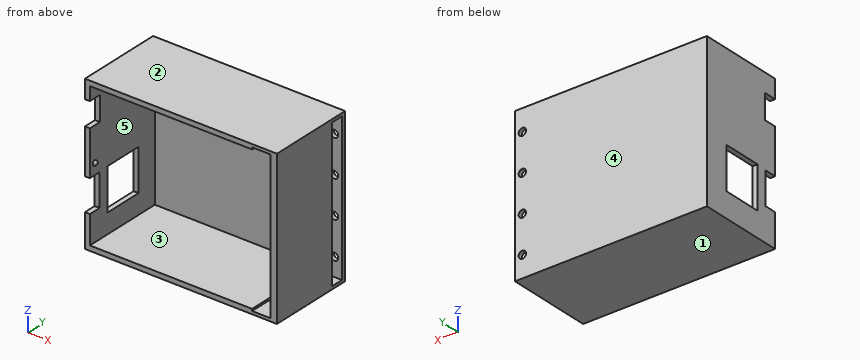
```python
from build123d import *

# Parameters (mm, degrees)
SKETCH1_W           = 77.9
SKETCH1_H           = 62.4
BOSS_EXTRUDE1_DEPTH = 35
SKETCH4_W           = 73.9
SKETCH4_H           = 58.4
CUT_EXTRUDE1_DEPTH  = 33.39
SKETCH7_W           = 13.133474477
SKETCH7_H           = 5
CUT_EXTRUDE6_DEPTH  = 15
SKETCH11_W          = 9.956525523
SKETCH11_H          = 5.15
CUT_EXTRUDE8_DEPTH  = 10
SKETCH12_W          = 17
SKETCH12_H          = 16
CUT_EXTRUDE9_DEPTH  = 10
SKETCH14_W          = 60
SKETCH14_H          = 5
CUT_EXTRUDE10_DEPTH = 10
CUT_EXTRUDE12_START = -33.39
SKETCH16_W          = 9.076585482
SKETCH16_H          = 60
CUT_EXTRUDE12_DEPTH = 33.39
SKETCH15_R          = 1.5
CUT_EXTRUDE11_DEPTH = 10
SKETCH18_W          = 1.605745829
SKETCH18_H          = 60
BOSS_EXTRUDE2_DEPTH = 10


with BuildPart() as part:
    # Sketch1 → Boss-Extrude1 (new body)
    with BuildSketch(Plane(origin=(0, 0, 0), x_dir=(1, 0, 0), z_dir=(0, 1, 0))):
        with Locations((38.95, 31.2)):
            Rectangle(SKETCH1_W, SKETCH1_H)
    extrude(amount=BOSS_EXTRUDE1_DEPTH)

    # Sketch4 → Cut-Extrude1 (cut)
    with BuildSketch(Plane.XZ):
        with Locations((38.95, -31.2)):
            Rectangle(SKETCH4_W, SKETCH4_H)
    extrude(amount=-CUT_EXTRUDE1_DEPTH, mode=Mode.SUBTRACT)

    # Sketch7 → Cut-Extrude6 (cut)
    with BuildSketch(Plane.ZY):
        with Locations((-42.333262762, 2.5)):
            Rectangle(SKETCH7_W, SKETCH7_H)
    extrude(amount=-CUT_EXTRUDE6_DEPTH, mode=Mode.SUBTRACT)

    # Sketch11 → Cut-Extrude8 (cut)
    with BuildSketch(Plane.ZY):
        with Locations((-12.508262762, 2.575)):
            Rectangle(SKETCH11_W, SKETCH11_H)
    extrude(amount=-CUT_EXTRUDE8_DEPTH, mode=Mode.SUBTRACT)

    # Sketch12 → Cut-Extrude9 (cut)
    with BuildSketch(Plane.ZY):
        with Locations((-43.9, 17)):
            Rectangle(SKETCH12_W, SKETCH12_H)
    extrude(amount=-CUT_EXTRUDE9_DEPTH, mode=Mode.SUBTRACT)

    # Sketch14 → Cut-Extrude10 (cut)
    with BuildSketch(Plane(origin=(77.9, 0, 0), x_dir=(0, 0, -1), z_dir=(1, 0, 0))):
        with Locations((31.2, 30.89)):
            Rectangle(SKETCH14_W, SKETCH14_H)
    extrude(amount=-CUT_EXTRUDE10_DEPTH, mode=Mode.SUBTRACT)

    # Sketch16 → Cut-Extrude12 (cut)
    with BuildSketch(Plane(origin=(0, 0, 0), x_dir=(-1, 0, 0), z_dir=(0, -1, 0)).offset(CUT_EXTRUDE12_START)):
        with Locations((-72.361707259, 31.2)):
            Rectangle(SKETCH16_W, SKETCH16_H)
    extrude(amount=CUT_EXTRUDE12_DEPTH, mode=Mode.SUBTRACT)

    # Sketch15 → Cut-Extrude11 (cut)
    with BuildSketch(Plane(origin=(0, 33.39, 0), x_dir=(-1, 0, 0), z_dir=(0, -1, 0))):
        with Locations(Location((-74.9, 8.7, 0), (0, 0, 90))):
            Circle(SKETCH15_R)
        with Locations(Location((-74.9, 23.7, 0), (0, 0, 90))):
            Circle(SKETCH15_R)
        with Locations(Location((-74.9, 38.7, 0), (0, 0, 90))):
            Circle(SKETCH15_R)
        with Locations(Location((-74.9, 53.7, 0), (0, 0, 90))):
            Circle(SKETCH15_R)
    extrude(amount=-CUT_EXTRUDE11_DEPTH, mode=Mode.SUBTRACT)

    # Sketch18 → Boss-Extrude2 (add)
    with BuildSketch(Plane(origin=(0, 0, 0), x_dir=(-1, 0, 0), z_dir=(0, -1, 0))):
        with Locations((-76.097127086, 31.2)):
            Rectangle(SKETCH18_W, SKETCH18_H)
    extrude(amount=-BOSS_EXTRUDE2_DEPTH)

    # Sketch19 → Revolve2 (revolve)
    with BuildSketch(Plane.ZY.offset(-75.294254171)):
        with BuildLine():
            Line((-31.2, 3.5), (-31.2, 1.5))
            ThreePointArc((-31.2, 1.5), (-30.2, 2.5), (-31.2, 3.5))
        make_face()
    revolve(axis=Axis((75.294254171, 3.5, -31.2), (0, -1, 0)))

    # Sketch17 → Revolve4 (revolve)
    with BuildSketch(Plane.ZY.offset(-2)):
        with BuildLine():
            ThreePointArc((-31.2, 3.5), (-32.2, 2.5), (-31.2, 1.5))
            Line((-31.2, 1.5), (-31.2, 3.5))
        make_face()
    revolve(axis=Axis((2, 3.5, -31.2), (0, -1, 0)))


solid = part.part
```
Geometry check sheet. Reference: the model listing, model coordinates, mm. Face numbers are marked on the shaded views. A direction names the side the tool comes from. Round coordinates to 2 decimals unless told otherwise and drop trailing zeros. Loops run counter-clockwise (first coordinate to the right, second up) from the corner with the lowest first, then second, coordinate; pieces in that order, holes last. Notation, with made-up numbers: (73.25, -31.75) - (91.25, -31.75) arc R20 ccw to (91.25, 7.25) - close; hole circle Ø4 at (42, 31.25). An arc over 180 degrees is marked (long way). Use a Markdown table: item, result.
Q1. Cross-section at B-B on z = -8.7. Record the cut outline in (x, y).
Solutions:
| item | result |
|---|---|
| outline | (0, 5.15) - (2, 5.15) - (2, 33.39) - (73.4, 33.39) - (73.4, 35) - (0, 35) - close; (75.29, 0) - (77.9, 0) - (77.9, 28.39) - (76.9, 28.39) - (76.9, 10) - (75.29, 10) - close; (76.4, 33.39) - (77.9, 33.39) - (77.9, 35) - (76.4, 35) - close |
Q2. Draft check along Z on the marked faces 1, 2 and 3. Enter one of: released by +Z, released by -Z, zero draft, split by the parting line, or undercut.
Solutions:
| item | result |
|---|---|
| face 1 | released by -Z |
| face 2 | released by +Z |
| face 3 | undercut |
Q3. Access from +Z, -Z, +X, -X, +Y, -Y to the whole of each face (thin tool, end or side, straight path). Record for the marked faces 4 and 5.
Solutions:
| item | result |
|---|---|
| face 4 | +Z, -Z, +X, -X, +Y |
| face 5 | none |
Q4. Go/stop test with flat-tipped pins: P1, Ø1, axis at x = 48.5, z = -12.5, coming from the -Y side; P2, Ø0.6, axis at x = 1.5, z = -44.5, coming from the -Y side; P3, Ø1.6, axis at x = 1.5, z = -13, coming from the -Y side. Record where each tip stops, or that it passes through.
Solutions:
| item | result |
|---|---|
| P1 | stops at y = 33.39 |
| P2 | stops at y = 5 |
| P3 | stops at y = 5.15 |
Q5. Cross-section at C-C on y = 29.5. Record the cut outline in (x, z).
Solutions:
| item | result |
|---|---|
| outline | (0, -62.4) - (77.9, -62.4) - (77.9, -61.2) - (67.82, -61.2) - (67.82, -60.4) - (2, -60.4) - (2, -2) - (67.82, -2) - (67.82, -1.2) - (77.9, -1.2) - (77.9, 0) - (0, 0) - close |
Q6. Material ranges on line 1 (Z direction, x = 74.9, y = 34.15); line 2 (Z direction, x = 71, y = 27.5); line 3 (X direction, y = 25.5, z = -57.5), recorded low to high.
Solutions:
| item | result |
|---|---|
| line 1 | z = -62.4 to -55.2, -52.2 to -40.2, -37.2 to -25.2, -22.2 to -10.2, -7.2 to 0 |
| line 2 | z = -62.4 to -61.2, -1.2 to 0 |
| line 3 | x = 0 to 2, 76.9 to 77.9 |
Q7. Cross-section at A-A on z = -38.7. Record the cut outline in (x, y).
Solutions:
| item | result |
|---|---|
| outline | (0, 5) - (2, 5) - (2, 9) - (0, 9) - close; (0, 25) - (2, 25) - (2, 33.39) - (73.4, 33.39) - (73.4, 35) - (0, 35) - close; (75.29, 0) - (77.9, 0) - (77.9, 28.39) - (76.9, 28.39) - (76.9, 10) - (75.29, 10) - close; (76.4, 33.39) - (77.9, 33.39) - (77.9, 35) - (76.4, 35) - close |
Q8. Cross-section at D-D on x = 10. Record the cut outline in (y, z), plus the area to 3 significant figures.
Solutions:
| item | result |
|---|---|
| outline | (0, -62.4) - (35, -62.4) - (35, 0) - (0, 0) - (0, -2) - (33.39, -2) - (33.39, -60.4) - (0, -60.4) - close |
| area | 234 mm2 |
